from build123d import *

# Parameters (mm, degrees)
F1_DEPTH = 19.05


with BuildPart() as f1:
    # F0 (on Right) → F1 (new body)
    with BuildSketch(Plane.YZ):
        with BuildLine():
            ThreePointArc((-6.35, 0), (0, 6.35), (6.35, 0))
            Line((6.35, 0), (6.725732, 0))
            Line((6.725732, 0), (6.725732, 76.2))
            Line((6.725732, 76.2), (-6.35, 76.2))
            Line((-6.35, 76.2), (-6.35, 0))
        make_face()
        with BuildLine():
            Line((3.1115, 0), (6.35, 0))
            ThreePointArc((6.35, 0), (0, 6.35), (-6.35, 0))
            Line((-6.35, 0), (-3.1115, 0))
            ThreePointArc((-3.1115, 0), (0, 3.1115), (3.1115, 0))
        make_face()
        with BuildLine():
            ThreePointArc((-6.35, 0), (0, -6.35), (6.35, 0))
            Line((6.35, 0), (3.1115, 0))
            ThreePointArc((3.1115, 0), (0, -3.1115), (-3.1115, 0))
            Line((-3.1115, 0), (-6.35, 0))
        make_face()
    extrude(amount=F1_DEPTH)


solid = f1.part
Verification items for the finished model (mm, model axes). Give positions to 0.01 mm unless a question says otherwise; leave off trailing zeros. Order: outer loops, then holes, each group sorted by start corner. A loop starts at its lowest first (then second) coordinate and runs counter-clockwise, first axis right, second up. Notation, with made-up numbers: M 26.5,39.5 L 73.5,39.5 A27 cw 73.5,62.5 Z; hole C 29,74.25 d7. An arc over 180 degrees is marked long. Use one line per item in the form item = value. Start each with the question number.
Q1. Section check B-B (x = 14.5). Enter the section's corners in (y, z).
Q2. Section check A-A (y = 0). Enter the section's corners in (x, z).
Q3. Scan lines: line 1 along Z through (x, y) = (12, 0); line 2 along Z through (x, y) = (3, -1.75); line 3 along Z through (x, y) = (7.75, 3.25). Record each from-to range of solid material in increasing order. Write a range as [from, to].
Q4. Section check C-C (y = -4.75). Enter the section's corners in (x, z).
Q5. Mould release check, pull along Y, two halves, no side actions. Record for faces 1 (the cylindrical face through (9.392, 2.874, 1.192)), 2 (the flat face through (19.05, 0, 36)), 3 (the cylindrical face through (9.39, -0.14, -6.35)): +Y half, -Y half, draft (parallel to the pull), parting line (faces both ways), or undercut.
Evaluation:
q1.outline = M -6.35,0 A6.35 ccw 6.35,0 L 6.73,0 L 6.73,76.2 L -6.35,76.2 Z; hole C 0,0 d6.22
q2.outline = M 0,-6.35 L 19.05,-6.35 L 19.05,-3.11 L 0,-3.11 Z; M 0,3.11 L 19.05,3.11 L 19.05,76.2 L 0,76.2 Z
q3.line_1 = [-6.35, -3.11], [3.11, 76.2]
q3.line_2 = [-6.1, -2.57], [2.57, 76.2]
q3.line_3 = [-5.46, 76.2]
q4.outline = M 0,-4.21 L 19.05,-4.21 L 19.05,76.2 L 0,76.2 Z
q5.face_1 = undercut
q5.face_2 = draft
q5.face_3 = parting line
